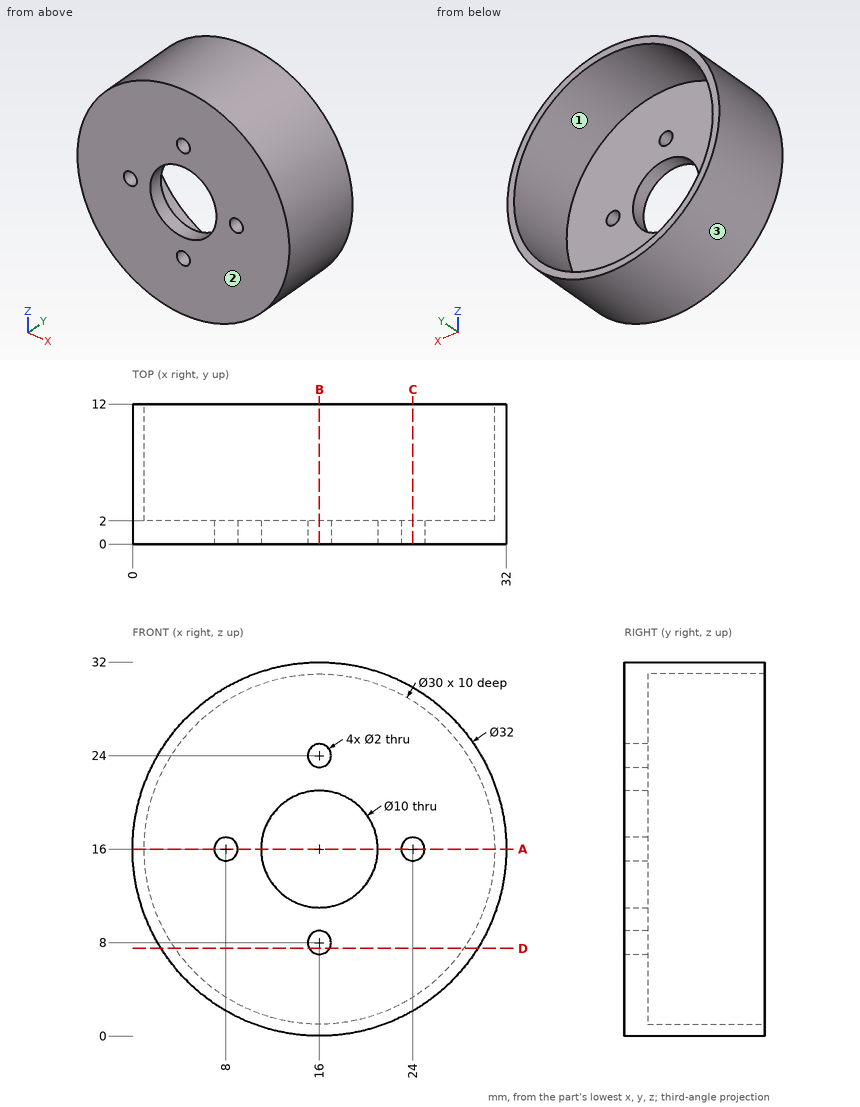
Here's the drawing with two shaded views (mm, measured from the low corner). I have some questions. Give positions to 0.01 mm unless a question says otherwise; leave off trailing zeros. Write each loop counter-clockwise with the first axis right and the second up, starting at its lowest first coordinate (ties: lowest second). Pieces come first, ordered by that corner, then holes. Notation, with made-up numbers: (25, -27.5) - (72, -27.5) arc R17 cw to (72, 3.5) - close; hole circle Ø1 at (-26, 76). An arc over 180 degrees is marked (long way). One line per item, written item: value. Start each with the question number.
Item 1: I'm going to push flat-ended pins straight in: pin 1 (13 mm diameter, centred on x = 16, z = 16, fed in from +Y); pin 2 (2 mm diameter, centred on x = 14, y = 3.5, fed in from -Z); pin 3 (1 mm diameter, centred on y = 8.5, z = 14.5, fed in from +X); pin 4 (1.6 mm diameter, centred on x = 16, z = 24, fed in from -Y). Where does each tip first touch, or does it pass through?
Item 2: Imagine slicing it at D-D, the plane z = 7.5. List the corners of the cut face in (x, y) for me, and give its area (3 significant figures).
Item 3: Imagine slicing it at B-B, the plane x = 16. List the corners of the cut face in (y, z) for me.
Item 4: Imagine slicing it at C-C, the plane x = 24. List the corners of the cut face in (y, z) for me, and give its area (3 significant figures).
Item 5: Please list where these lines run through material, in increasing order: line 1 (X direction, y = 0.95, z = 16); line 2 (Z direction, x = 16.5, y = 1.25); line 3 (X direction, y = 5, z = 16). Write a range as from..to.
Item 6: Imagine slicing it at A-A, the plane z = 16. List the corners of the cut face in (x, y) for me.
Item 7: If we mould it in two halves opening along Z, with no side actions, what happens to the marked faces 1, 2 and 3? For each: +Z half, -Z half, draft (parallel to the pull), parting line (faces both ways), or undercut.
Geometry says:
1. pin 1: y = 2
1. pin 2: z = 0.03
1. pin 3: x = 31.97
1. pin 4: through
2. outline: (2.44, 0) - (15.13, 0) - (15.13, 2) - (3.64, 2) - (3.64, 12) - (2.44, 12) - close; (16.87, 0) - (29.56, 0) - (29.56, 12) - (28.36, 12) - (28.36, 2) - (16.87, 2) - close
2. area: 74.7 mm^2
3. outline: (0, 0) - (12, 0) - (12, 1) - (2, 1) - (2, 7) - (0, 7) - close; (0, 9) - (2, 9) - (2, 11) - (0, 11) - close; (0, 21) - (2, 21) - (2, 23) - (0, 23) - close; (0, 25) - (2, 25) - (2, 31) - (12, 31) - (12, 32) - (0, 32) - close
4. outline: (0, 2.14) - (12, 2.14) - (12, 3.31) - (2, 3.31) - (2, 15) - (0, 15) - close; (0, 17) - (2, 17) - (2, 28.69) - (12, 28.69) - (12, 29.86) - (0, 29.86) - close
4. area: 74.8 mm^2
5. line 1: 0..7, 9..11, 21..23, 25..32
5. line 2: 0.01..7.13, 8.87..11.03, 20.97..23.13, 24.87..31.99
5. line 3: 0..1, 31..32
6. outline: (0, 0) - (7, 0) - (7, 2) - (1, 2) - (1, 12) - (0, 12) - close; (9, 0) - (11, 0) - (11, 2) - (9, 2) - close; (21, 0) - (23, 0) - (23, 2) - (21, 2) - close; (25, 0) - (32, 0) - (32, 12) - (31, 12) - (31, 2) - (25, 2) - close
7. face 1: undercut
7. face 2: draft
7. face 3: parting line
